Answer from the drawing. Dimensions are ordinates in mm from the lowest x, y and z of the part. A direction names the side the tool comes from. Give positions to 0.01 mm unless a question says otherwise; leave off trailing zeros. Order: outer loops, then holes, each group sorted by start corner. A loop starts at its lowest first (then second) coordinate and runs counter-clockwise, first axis right, second up. Notation, with made-up numbers: (-5, 50) - (50, 50) arc R27 ccw to (50, 75) - close; hole circle Ø7 at (32.25, -14). An arc over 180 degrees is marked (long way). Use a Markdown table: item, result. Add a question column.
1) Find section C-C, the plane z = 63. Determine the outline of the cut face in (x, y), plus the area to 3 significant figures.
2) Flat-ended cylindrical pins translate along their axes: pin 1 (3 mm diameter, centred on x = 11, y = 66, fed in from +Z); pin 2 (8 mm diameter, centred on x = 13.5, z = 9.5, fed in from +Y); pin 3 (4 mm diameter, centred on x = 5.5, z = 73, fed in from -Y); pin 4 (8 mm diameter, centred on y = 23.5, z = 20, fed in from -X). Find the tip coordinate at first contact, or state that the pin passes through.
3) Straight lines are drawn through the part: line 1 (Z direction, x = 16, y = 162.5); line 2 (Y direction, x = 3, z = 33.5) (1 decimal). For each, find the intervals that lie inside material, in ascending order.
4) For the marked faces 1 and 2, determine the directions among +Z, -Z, +X, -X, +Y, -Y from which every point of the face is accessible in a straight line to the end or side of a thin tool.
5) Find section D-D, the plane x = 14. Determine the outline of the cut face in (y, z).
6) Find section A-A, the plane z = 53. Determine the outline of the cut face in (x, y).
7) Find section B-B, the plane y = 48. Determine the outline of the cut face in (x, z).
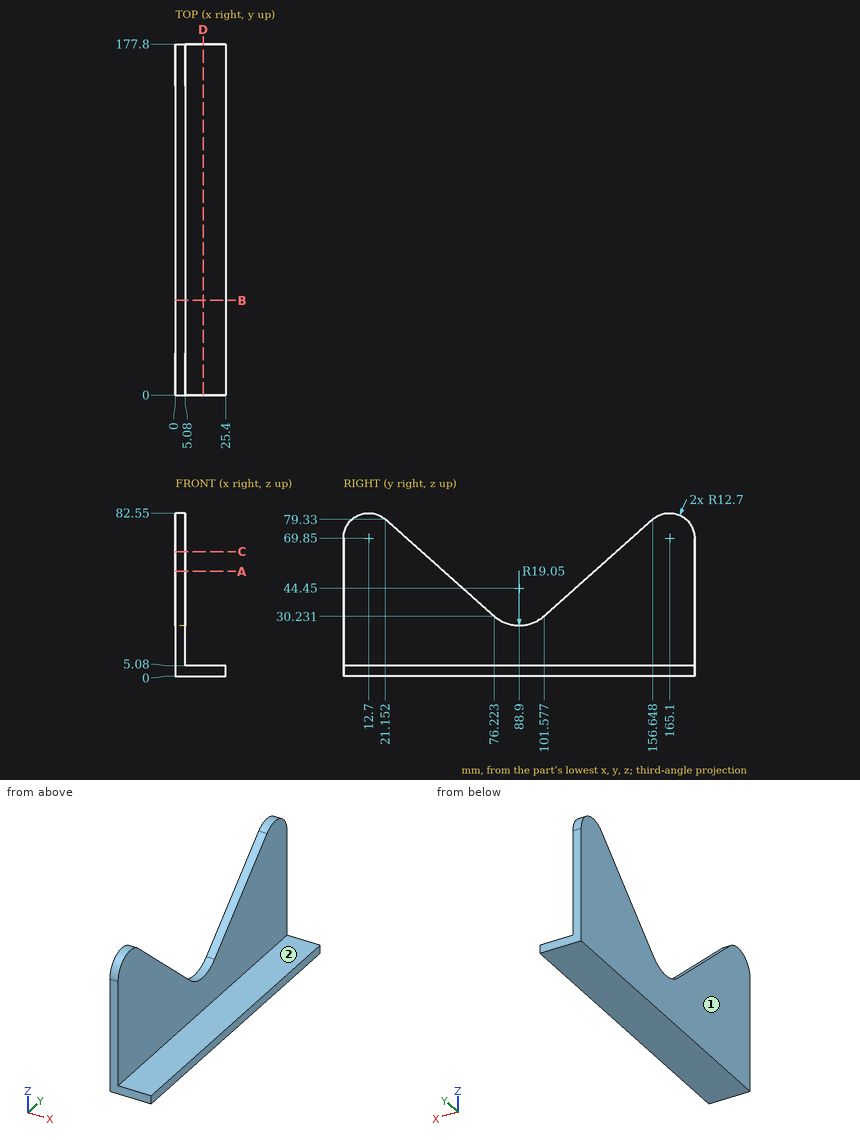
The answers:
| question | item | result |
|---|---|---|
| 1 | outline | (0, 0) - (5.08, 0) - (5.08, 39.47) - (0, 39.47) - close; (0, 138.33) - (5.08, 138.33) - (5.08, 177.8) - (0, 177.8) - close |
| 1 | area | 401 mm2 |
| 2 | pin 1 | z = 5.08 |
| 2 | pin 2 | through |
| 2 | pin 3 | y = 0.06 |
| 2 | pin 4 | x = 0 |
| 3 | line 1 | 0 to 5.08 |
| 3 | line 2 | 0 to 72.6, 105.2 to 177.8 |
| 4 | face 1 | +Z, -Z, -X, +Y, -Y |
| 4 | face 2 | +Z, +X, +Y, -Y |
| 5 | outline | (0, 0) - (177.8, 0) - (177.8, 5.08) - (0, 5.08) - close |
| 6 | outline | (0, 0) - (5.08, 0) - (5.08, 50.68) - (0, 50.68) - close; (0, 127.12) - (5.08, 127.12) - (5.08, 177.8) - (0, 177.8) - close |
| 7 | outline | (0, 0) - (25.4, 0) - (25.4, 5.08) - (5.08, 5.08) - (5.08, 55.39) - (0, 55.39) - close |
